```python
from build123d import *

# Parameters (mm, degrees)
F2_DEPTH = 4.8514
F3_R     = 4.85139
F4_R     = 1.397
F5_DEPTH = 25.4


# Not quite as in the source:
# - a variable given as a bare number and used for a length is read in inches; the dataset says mm whatever the document's units were
# - a fillet or chamfer is up to 0.001 mm smaller than in the source, because OpenCascade refuses the exact size


with BuildPart() as f2:
    # F1 (on Front) → F2 (new body, symmetric)
    with BuildSketch(Plane.XZ):
        with BuildLine():
            ThreePointArc((-7.5137404391, 8.2587754484), (-5.3542263452, 2.6761311983), (0, 0))
            Line((0, 0), (34.9550595609, 0))
            Line((34.9550595609, 0), (34.9550595609, 2.9464))
            Line((34.9550595609, 2.9464), (0, 2.9464))
            ThreePointArc((0, 2.9464), (-3.271499032, 4.6780426472), (-4.5800404391, 8.1405578545))
            Line((-4.5800404391, 8.1405578545), (-4.5800404391, 19.177))
            Line((-4.5800404391, 19.177), (-7.5137404391, 19.177))
            Line((-7.5137404391, 19.177), (-7.5137404391, 8.2587754484))
        make_face()
    extrude(amount=F2_DEPTH, both=True)

    # F3 (radius 4.8514 in the source; OpenCascade refuses exactly that, so slightly less here)
    f3_edges = [f2.edges().sort_by_distance(p)[0] for p in [
        (34.95506, -4.8514, 1.4732),
        (34.95506, 4.8514, 1.4732),
        (-6.04689, -4.8514, 19.177),
        (-6.04689, 4.8514, 19.177),
    ]]
    fillet(f3_edges, radius=F3_R)

    # F4 (on face) → F5 (cut)
    with BuildSketch(Plane.XY.offset(2.9464)):
        with Locations((30.1036595609, 0)):
            Circle(F4_R)
    extrude(amount=-F5_DEPTH, mode=Mode.SUBTRACT)


solid = f2.part
```
Verification items for the finished model (mm, model axes). A direction names the side the tool comes from. Give positions to 0.01 mm unless a question says otherwise; leave off trailing zeros. Order: outer loops, then holes, each group sorted by start corner. A loop starts at its lowest first (then second) coordinate and runs counter-clockwise, first axis right, second up. Notation, with made-up numbers: M 3.5,7 L 43.5,7 A13 cw 43.5,29 Z; hole C -1.5,48 d9. An arc over 180 degrees is marked long. Return JSON: item names as keys, results as strings. Group by question number.
1) Access from +Z, -Z, +X, -X, +Y, -Y to the whole of each face (thin tool, end or side, straight path). Record for faces 1 (the face through (-4.58, 0, 14)), 2 (the face through (33.572, -3.393, 1.494)).
2) Go/stop test with flat-tipped pins: pin 1 Ø5 at (x, z) = (13, 6.5) entering from -Y; pin 2 Ø4 at (x, y) = (26, -0.5) entering from +Z. Record where each tip stops, or that it passes through.
3) Section check D-D on x = 2.5. Record the cut outline in (y, z), and give its area (3 significant figures).
4) Section check C-C on y = 2.75. Record the cut outline in (x, z).
5) Mould release check, pull along X, two halves, no side actions. Record for faces 3 (the face through (31.436, 0.42, 1.494)), 4 (the face through (-6.067, -3.393, 17.794)), 5 (the face through (33.572, 3.393, 1.494)): pulls with the +X half, pulls with the -X half, needs draft (parallel to the pull), parting line crosses it, or undercut.
6) Section check B-B on y = 1. Record the cut outline in (x, z).
7) Scan lines: line 1 (X direction, y = 4, z = 16.25); line 2 (Z direction, x = 2.5, y = 0.5); line 3 (Z direction, x = -2, y = -3). Record each from-to range of solid material in increasing order.
Answer block:
{
 "1": {"face 1": "+Z, +X, +Y, -Y", "face 2": "+Z, -Z, +X, -Y"},
 "2": {"pin 1": "passes through", "pin 2": "stops at z = 2.95"},
 "3": {"outline": "M -4.85,0 L 4.85,0 L 4.85,2.95 L -4.85,2.95 Z", "area": "28.6 mm^2"},
 "4": {"outline": "M -7.51,8.26 A8.3 ccw 0,0 L 34.1,0 L 34.1,2.95 L 0,2.95 A5.24 cw -4.58,8.14 L -4.58,18.32 L -7.51,18.32 Z"},
 "5": {"face 3": "undercut", "face 4": "needs draft", "face 5": "pulls with the +X half"},
 "6": {"outline": "M -7.51,8.26 A8.3 ccw 0,0 L 29.13,0 L 29.13,2.95 L 0,2.95 A5.24 cw -4.58,8.14 L -4.58,19.07 L -7.51,19.07 Z; M 31.08,0 L 34.85,0 L 34.85,2.95 L 31.08,2.95 Z"},
 "7": {"line 1": "x = -7.51 to -4.58", "line 2": "z = 0 to 2.95", "line 3": "z = 0.44 to 3.63"}
}
